Build history of the part. All positions in model axes, mm. Give positions to 0.01 mm unless a question says otherwise; leave off trailing zeros. Write each loop counter-clockwise with the first axis right and the second up, starting at its lowest first coordinate (ties: lowest second). Pieces come first, ordered by that corner, then holes. Notation, with made-up numbers: M -27,-38 L 15,-38 A11 ccw 15,-19 Z; hole C 21.5,-14.5 d10. An arc over 180 degrees is marked long. Return JSON: item names as keys, results as strings. Group by question number.
Q1. Band-saw the part on C-C, the plane x = 26.5. Give the cut face in (y, z).
Q2. Band-saw the part on D-D, the plane x = 20.5. Give the cut face in (y, z).
Q3. Flat gauge pins, fed straight in: pin 1 Ø0.5 at (y, z) = (78.5, 0.5) entering from +X; pin 2 Ø1.4 at (x, y) = (3.02, -5.72) entering from +Z. Where does each tip first touch, or does it go through?
Q4. Band-saw the part on B-B, the plane z = 0.55. Give the cut face in (x, y).
Q5. Wall check: probe 1 along Y at (x, z) = (31.75, 0.4); probe 2 along Y at (x, z) = (29.5, 0.25); probe 3 along X at (y, z) = (80, 0.25). Give the ranges that are in metal, low to high.
Q6. Band-saw the part on A-A, the plane x = 31.75. Give the cut face in (y, z), then the cut area to 3 significant figures.
from build123d import *

# Parameters (mm, degrees)
SKETCH1_W                  = 19.05
SKETCH1_H                  = 88.9
BOSS_EXTRUDE1_DEPTH        = 1.5875
SKETCH4_W                  = 21.59
SKETCH4_H                  = 71.755
BOSS_EXTRUDE2_DEPTH        = 1.5875
CHAMFER1_SIZE              = 10
SKETCH5_W                  = 40.64
SKETCH5_H                  = 2.54
SKETCH5_W_2                = 19.05
SKETCH5_H_2                = 1.5875
BOSS_EXTRUDE3_DEPTH        = 1.5875
F_2_3_2_3_DIAMETER_HOLE1_D = 2.3


with BuildPart() as part:
    # Sketch1 → Boss-Extrude1 (new body)
    with BuildSketch(Plane.XY):
        with Locations((3.01625, 39.14175)):
            Rectangle(SKETCH1_W, SKETCH1_H)
    extrude(amount=BOSS_EXTRUDE1_DEPTH)

    # Sketch4 → Boss-Extrude2 (add, through all)
    with BuildSketch(Plane.XY.offset(1.5875)):
        with Locations((23.33625, 30.56925)):
            Rectangle(SKETCH4_W, SKETCH4_H)
    extrude(amount=-BOSS_EXTRUDE2_DEPTH)

    # Chamfer1
    chamfer1_edges = [part.edges().sort_by_distance(p)[0] for p in [
        (12.54125, 66.44675, 0.79375),
    ]]
    chamfer(chamfer1_edges, length=CHAMFER1_SIZE)

    # Sketch5 → Boss-Extrude3 (add, through all)
    with BuildSketch(Plane.XY.offset(1.5875)):
        with Locations((13.81125, -6.57825)):
            Rectangle(SKETCH5_W, SKETCH5_H)
        with Locations((3.01625, 84.3855)):
            Rectangle(SKETCH5_W_2, SKETCH5_H_2)
    extrude(amount=-BOSS_EXTRUDE3_DEPTH)

    # Ø2.3 (2.3) Diameter Hole1 (through all)
    with Locations(Plane.XY.offset(1.5875)):
        with Locations((14.9225, 45.1655), (31.75, 64.0655), (31.75, -5.467), (3.01625, -5.721)):
            Hole(F_2_3_2_3_DIAMETER_HOLE1_D / 2)


solid = part.part
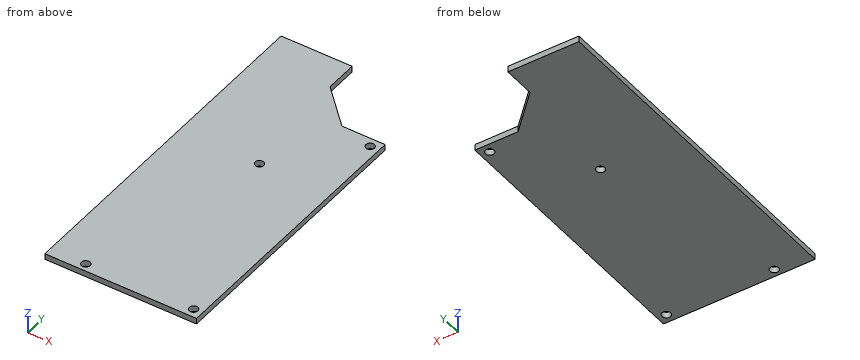
From the geometry:
{
 "1": {"outline": "M -7.85,0 L 66.45,0 L 66.45,1.59 L -7.85,1.59 Z"},
 "2": {"outline": "M -7.85,0 L 68.49,0 L 68.49,1.59 L -7.85,1.59 Z"},
 "3": {"pin 1": "stops at x = 12.54", "pin 2": "passes through"},
 "4": {"outline": "M -6.51,-7.85 L 34.13,-7.85 L 34.13,66.45 L 22.54,66.45 L 12.54,76.45 L 12.54,85.18 L -6.51,85.18 Z; hole C 3.02,-5.72 d2.3; hole C 14.92,45.17 d2.3; hole C 31.75,-5.47 d2.3; hole C 31.75,64.07 d2.3"},
 "5": {"probe 1": "y = -7.85 to -6.62, -4.32 to 62.92, 65.22 to 66.45", "probe 2": "y = -7.85 to 66.45", "probe 3": "x = -6.51 to 12.54"},
 "6": {"outline": "M -7.85,0 L -6.62,0 L -6.62,1.59 L -7.85,1.59 Z; M -4.32,0 L 62.92,0 L 62.92,1.59 L -4.32,1.59 Z; M 65.22,0 L 66.45,0 L 66.45,1.59 L 65.22,1.59 Z", "area": "111 mm^2"}
}
